Check sheet for the modelled part. Datum: model origin and axes. Units: mm. Round coordinates to 2 decimals unless told otherwise and drop trailing zeros. Order: outer loops, then holes, each group sorted by start corner. A loop starts at its lowest first (then second) coordinate and runs counter-clockwise, first axis right, second up.
Q1. Cross-section at C-C on z = 7.25. Record the cut outline in (x, y), then the cut area to 3 significant figures.
Q2. Cross-section at B-B on x = -18.5. Record the cut outline in (y, z).
Q3. Scan lines: probe 1 along X at (y, z) = (0, 6.5); probe 2 along Y at (x, z) = (-30, 7). Record each from-to range of solid material in increasing order.
Q4. Depth check by flat-ended pin: P1, Ø7, axis at x = 31.47, y = 31.47, coming from the -Z side. Enter the tip coordinate at first touch or a pass-through.
Q5. Mould release check, pull along X, two halves, no side actions. Record for faces 1 (the flat face through (0, 41.5, 5)), 2 (the cylindrical face through (29.681, -32.835, 4.93)), 3 (the flat face through (-29.09, -38.47, 4.93)), 4 (the cylindrical face through (-8.67, -39.05, 4.93)): +X half, -X half, draft (parallel to the pull), parting line (faces both ways), or undercut.
Q6. Cross-section at A-A on y = 0. Record the cut outline in (x, z).
from build123d import *

# Parameters (mm, degrees)
PAD_DEPTH    = 10
SKETCH_R     = 40
SKETCH_R_2   = 2.25
POCKET_DEPTH = 10.001


with BuildPart() as part:
    # Sketch001 → Pad (new body)
    with BuildSketch(Plane.XY):
        Polygon((-23, 41.5), (23, 41.5), (35.355339, 35.355339), (41.5, 23), (41.5, -23), (35.355339, -35.355339), (23, -41.5), (-23, -41.5), (-35.355339, -35.355339), (-41.5, -23), (-41.5, 23), (-35.355339, 35.355339), align=None)
    extrude(amount=PAD_DEPTH)

    # Sketch → Pocket (cut, through all)
    with BuildSketch(Plane.XY):
        Circle(SKETCH_R)
        with Locations((31.466252, 31.466252)):
            Circle(SKETCH_R_2)
        with Locations((-31.466252, 31.466252)):
            Circle(SKETCH_R_2)
        with Locations((31.466252, -31.466252)):
            Circle(SKETCH_R_2)
        with Locations((-31.466252, -31.466252)):
            Circle(SKETCH_R_2)
    extrude(amount=POCKET_DEPTH, mode=Mode.SUBTRACT)


solid = part.part
Results found:
1. outline: (-41.5, -23) - (-35.36, -35.36) - (-23, -41.5) - (23, -41.5) - (35.36, -35.36) - (41.5, -23) - (41.5, 23) - (35.36, 35.36) - (23, 41.5) - (-23, 41.5) - (-35.36, 35.36) - (-41.5, 23) - close; hole circle Ø80 at (0, 0); hole circle Ø4.5 at (-31.47, -31.47); hole circle Ø4.5 at (-31.47, 31.47); hole circle Ø4.5 at (31.47, -31.47); hole circle Ø4.5 at (31.47, 31.47)
1. area: 1,340 mm2
2. outline: (-41.5, 0) - (-35.46, 0) - (-35.46, 10) - (-41.5, 10) - close; (35.46, 0) - (41.5, 0) - (41.5, 10) - (35.46, 10) - close
3. probe 1: x = -41.5 to -40, 40 to 41.5
3. probe 2: y = -38.02 to -33.17, -29.76 to -26.46, 26.46 to 29.76, 33.17 to 38.02
4. P1: stops at z = 0
5. face 1: draft
5. face 2: undercut
5. face 3: -X half
5. face 4: undercut
6. outline: (-41.5, 0) - (-40, 0) - (-40, 10) - (-41.5, 10) - close; (40, 0) - (41.5, 0) - (41.5, 10) - (40, 10) - close
